Geometry check sheet. Reference: the model listing, model coordinates, mm. Face numbers are marked on the shaded views. Coordinates: 2 decimals unless noted, no trailing zeros. Order: outer loops, then holes, each group sorted by start corner. A loop starts at its lowest first (then second) coordinate and runs counter-clockwise, first axis right, second up. Notation, with made-up numbers: (56.5, 26) -> (68.5, 26) arc R19 ccw to (68.5, 52) -> close; hole circle Ø8 at (31.5, 45). An arc over 180 degrees is marked (long way). Answer in a Markdown table with one row per item. Add a question column.
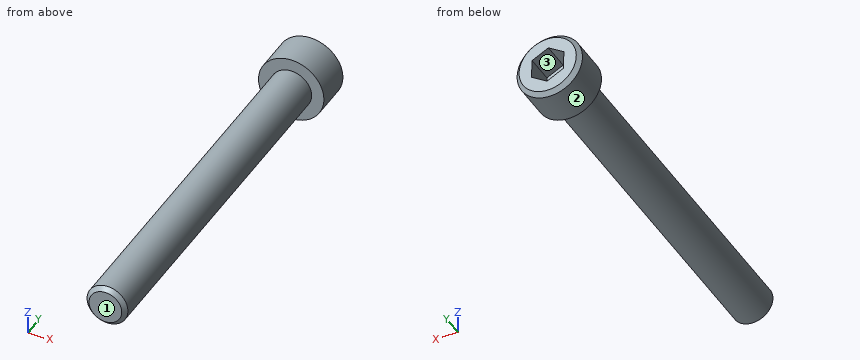
```python
from build123d import *

# Parameters (mm, degrees)
SKETCH1_R           = 5
BOSS_EXTRUDE1_DEPTH = 88
SKETCH2_R           = 8
BOSS_EXTRUDE2_DEPTH = 10
CUT_EXTRUDE1_DEPTH  = 7


with BuildPart() as part:
    # Sketch1 → Boss-Extrude1 (new body)
    with BuildSketch(Plane(origin=(0, 0, 0), x_dir=(1, 0, 0), z_dir=(0, 1, 0))):
        with Locations(Location((0, 0, 0), (0, 0, 270))):
            Circle(SKETCH1_R)
    extrude(amount=BOSS_EXTRUDE1_DEPTH)

    # Sketch2 → Boss-Extrude2 (add)
    with BuildSketch(Plane(origin=(0, 88, 0), x_dir=(1, 0, 0), z_dir=(0, 1, 0))):
        with Locations(Location((0, 0, 0), (0, 0, 270))):
            Circle(SKETCH2_R)
    extrude(amount=BOSS_EXTRUDE2_DEPTH)

    # Sketch3 → Cut-Revolve1 (revolve, cut)
    with BuildSketch(Plane.XY, mode=Mode.PRIVATE) as cut_revolve1_sk:
        Polygon((8, 98), (8, 97), (7, 98), align=None)
    revolve(cut_revolve1_sk.sketch.rotate(Axis((0, 98, 0), (0, -1, 0)), 90), axis=Axis((0, 98, 0), (0, -1, 0)), mode=Mode.SUBTRACT)

    # Sketch4 → Cut-Revolve2 (revolve, cut)
    with BuildSketch(Plane.XY, mode=Mode.PRIVATE) as cut_revolve2_sk:
        Polygon((5, 0), (4, 0), (5, 1), align=None)
    revolve(cut_revolve2_sk.sketch.rotate(Axis((0, 0, 0), (0, 1, 0)), 90), axis=Axis((0, 0, 0), (0, 1, 0)), mode=Mode.SUBTRACT)

    # Sketch5 → Cut-Extrude1 (cut)
    with BuildSketch(Plane(origin=(0, 98, 0), x_dir=(1, 0, 0), z_dir=(0, 1, 0))):
        Polygon((-0.172380767, -4.496697107), (3.808063544, -2.397634677), (3.980444311, 2.09906243), (0.172380767, 4.496697107), (-3.808063544, 2.397634677), (-3.980444311, -2.09906243), align=None)
    extrude(amount=-CUT_EXTRUDE1_DEPTH, mode=Mode.SUBTRACT)


solid = part.part
```
(1) Go/stop test with flat-tipped pins: P1, Ø1, axis at x = 2, y = 70, coming from the +Z side; P2, Ø5, axis at x = -6.5, y = 49, coming from the +Z side; P3, Ø6, axis at y = 46, z = 5, coming from the +X side. Record where each tip stops, or that it passes through.
(2) Mould release check, pull along Z, two halves, no side actions. Record for the marked faces 1, 2 and 3: +Z half, -Z half, draft (parallel to the pull), parting line (faces both ways), or undercut.
(3) Scan lines: line 1 along Z through (x, y) = (3.25, 80.5); line 2 along X through (y, z) = (92, 3.25); line 3 along Y through (x, z) = (4.5, -3.25). Record each from-to range of solid material in increasing order.
(4) Cross-section at B-B (y = 63.5). Enter the section's corners in (x, z), plus the area to 3 significant figures.
(5) Cross-section at A-A (z = 0). Enter the section's corners in (x, y), plus the area to 3 significant figures.
Checks:
| question | item | result |
|---|---|---|
| 1 | P1 | z = 4.77 |
| 1 | P2 | z = 3 |
| 1 | P3 | x = 4.58 |
| 2 | face 1 | draft |
| 2 | face 2 | parting line |
| 2 | face 3 | undercut |
| 3 | line 1 | -3.8 to 3.8 |
| 3 | line 2 | -7.31 to -2.15, 2.19 to 7.31 |
| 3 | line 3 | 88 to 98 |
| 4 | outline | circle Ø10 at (0, 0) |
| 4 | area | 78.5 mm² |
| 5 | outline | (-8, 88) -> (-5, 88) -> (-5, 1) -> (-4, 0) -> (4, 0) -> (5, 1) -> (5, 88) -> (8, 88) -> (8, 97) -> (7, 98) -> (3.9, 98) -> (3.9, 91) -> (-3.9, 91) -> (-3.9, 98) -> (-7, 98) -> (-8, 97) -> close |
| 5 | area | 983 mm² |
